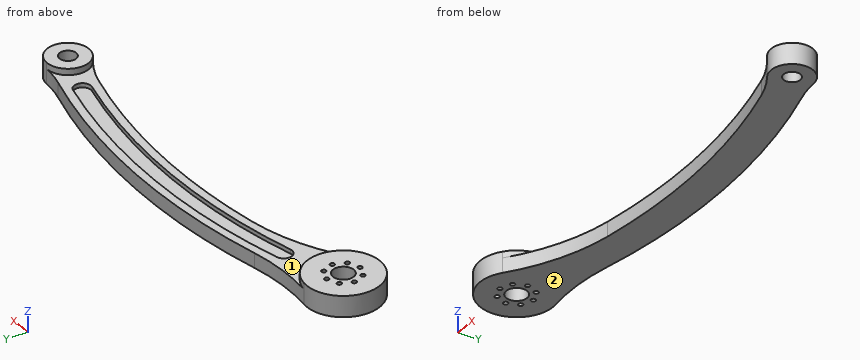
from build123d import *

# Parameters (mm, degrees)
SKETCH1_R                = 5
SKETCH1_R_2              = 4
BOSS_EXTRUDE1_DEPTH      = 10
FILLET1_R                = 100
FILLET3_R                = 50
BOSS_EXTRUDE2_DEPTH      = 5
CUT_EXTRUDE1_DEPTH       = 3
M2_CLEARANCE_HOLE2_D     = 2.2
M2_CLEARANCE_HOLE2_DEPTH = 10


with BuildPart() as part:
    # Sketch1 → Boss-Extrude1 (new body)
    with BuildSketch(Plane.XY):
        with BuildLine():
            ThreePointArc((12.332289397, 12.416305338), (-16.645203494, -5.40251799), (17.2733755, -2.807222621))
            ThreePointArc((17.2733755, -2.807222621), (104.699737116, 9.220908362), (191.757044964, -5.238337488))
            ThreePointArc((191.757044964, -5.238337488), (209.474645485, -2.773362317), (196.872940476, 9.922562291))
            ThreePointArc((196.872940476, 9.922562291), (104.792499107, 25.221141559), (12.332289397, 12.416305338))
        make_face()
        Circle(SKETCH1_R, mode=Mode.SUBTRACT)
        with Locations((199.999550741, 0.423914585)):
            Circle(SKETCH1_R_2, mode=Mode.SUBTRACT)
        with BuildLine():
            ThreePointArc((30.935149345, 4.991193321), (105.08187222, 13.215793431), (178.947951069, 2.766728612))
            ThreePointArc((178.947951069, 2.766728612), (183.85884318, 5.57442138), (181.051150412, 10.485313491))
            ThreePointArc((181.051150412, 10.485313491), (105.20208958, 21.214890117), (29.064850655, 12.769495373))
            ThreePointArc((29.064850655, 12.769495373), (26.110848974, 7.945195001), (30.935149345, 4.991193321))
        make_face(mode=Mode.SUBTRACT)
    extrude(amount=BOSS_EXTRUDE1_DEPTH)

    # Fillet1
    fillet1_edges = [part.edges().sort_by_distance(p)[0] for p in [
        (17.2733755, -2.807222621, 5),
        (12.332289397, 12.416305338, 5),
    ]]
    fillet(fillet1_edges, radius=FILLET1_R)

    # Fillet3
    fillet3_edges = [part.edges().sort_by_distance(p)[0] for p in [
        (196.872940476, 9.922562291, 5),
        (191.757044964, -5.238337488, 5),
    ]]
    fillet(fillet3_edges, radius=FILLET3_R)

    # Sketch2 → Boss-Extrude2 (add)
    with BuildSketch(Plane(origin=(0, 0, 0), x_dir=(-1, 0, 0), z_dir=(0, 0, -1))):
        with BuildLine():
            ThreePointArc((-30.935149345, 4.991193321), (-26.110848974, 7.945195001), (-29.064850655, 12.769495373))
            ThreePointArc((-29.064850655, 12.769495373), (-105.20208958, 21.214890117), (-181.051150412, 10.485313491))
            ThreePointArc((-181.051150412, 10.485313491), (-183.85884318, 5.57442138), (-178.947951069, 2.766728612))
            ThreePointArc((-178.947951069, 2.766728612), (-105.08187222, 13.215793431), (-30.935149345, 4.991193321))
        make_face()
    extrude(amount=-BOSS_EXTRUDE2_DEPTH)

    # Sketch3 → Cut-Extrude1 (cut)
    with BuildSketch(Plane.XY.offset(10)):
        with BuildLine():
            ThreePointArc((10.719889508, -13.832352256), (16.904607487, 4.525952466), (2.374455951, 17.338164809))
            ThreePointArc((2.374455951, 17.338164809), (19.536178227, 16.477975853), (36.591800033, 18.568526337))
            ThreePointArc((36.591800033, 18.568526337), (113.1236291, 24.996521405), (188.887012749, 12.412814518))
            ThreePointArc((188.887012749, 12.412814518), (194.644535138, 11.067035799), (200.520666376, 10.410327279))
            ThreePointArc((200.520666376, 10.410327279), (190.475667826, 3.472792121), (194.624244359, -8.008527607))
            ThreePointArc((194.624244359, -8.008527607), (188.279056755, -4.580565267), (181.506715916, -2.10110341))
            ThreePointArc((181.506715916, -2.10110341), (119.798948798, 8.622149082), (57.220022333, 6.030888954))
            ThreePointArc((57.220022333, 6.030888954), (32.693746361, -0.913106752), (10.719889508, -13.832352256))
        make_face()
    extrude(amount=-CUT_EXTRUDE1_DEPTH, mode=Mode.SUBTRACT)

    # M2 Clearance Hole2
    with Locations(Plane.XY.offset(10)):
        with Locations((0, 8), (5.656854249, 5.656854249), (8, 0), (5.656854249, -5.656854249), (0, -8), (-5.656854249, -5.656854249), (-8, 0), (-5.656854249, 5.656854249)):
            Hole(M2_CLEARANCE_HOLE2_D / 2, depth=M2_CLEARANCE_HOLE2_DEPTH)


solid = part.part
For this review, take the finished solid that the model builds, in its own axes (mm). Face numbers are marked on the shaded views. Round coordinates to 2 decimals unless told otherwise and drop trailing zeros. Order: outer loops, then holes, each group sorted by start corner. A loop starts at its lowest first (then second) coordinate and runs counter-clockwise, first axis right, second up. Notation, with made-up numbers: (-26, -9.5) -> (4, -9.5) arc R16 ccw to (4, 6.5) -> close; hole circle Ø10 at (26.5, -20.5). An arc over 180 degrees is marked (long way). Put each result on its own line as item: value.
Q1. Add section B-B on z = 2.75. State how many separate pieces and enclosed holes the cut face has, plus the area to 3 significant figures.
Check result:
separate pieces: 1
enclosed holes: 10
area: 4,110 mm2
Q2. Insertion check: pin 1 Ø1.5 at (x, z) = (146, 1.5) entering from -Y; pin 2 Ø1.8 at (x, y) = (-8, 0) entering from +Z; pin 3 Ø5 at (x, z) = (71.5, 4) entering from -Y; pin 4 Ø2 at (x, z) = (166.5, 5) entering from +Y. Each pin has a flat end and moves straight along its axis. Give the tip position at first contact, or say it passes through.
Check result:
pin 1: y = 5.61
pin 2: through
pin 3: y = 7.55
pin 4: y = 18.38
Q3. Add section A-A on x = 88.5. Write out the cut boundary in (y, z), plus the area to 3 significant figures.
Check result:
outline: (9, 0) -> (25.01, 0) -> (25.01, 7) -> (21.01, 7) -> (21.01, 5) -> (13, 5) -> (13, 7) -> (9, 7) -> close
area: 96.1 mm2
Q4. Mouldability with a two-part tool opening along X and no side actions: class the marked faces 1 and 2 as pulls with the +X half, pulls with the -X half, needs draft (parallel to the pull), parting line crosses it, or undercut.
Check result:
face 1: undercut
face 2: needs draft
Q5. Add section C-C on x = 115.5. Write out the cut boundary in (y, z), plus the area to 3 significant figures.
Check result:
outline: (8.87, 0) -> (24.89, 0) -> (24.89, 7) -> (20.89, 7) -> (20.89, 5) -> (12.88, 5) -> (12.88, 7) -> (8.87, 7) -> close
area: 96.1 mm2
Q6. For probe 1 along X at (y, z) = (-7, 4.5); probe 2 along Z at (x, y) = (148, 11.5); probe 3 along X at (y, z) = (7.5, 9), list the stretches that pass through material, from the lowest coordinate up. Write a range as [from, to].
Check result:
probe 1: [-16.04, -0.46], [0.46, 20.74], [192.97, 206.7]
probe 2: [0, 5]
probe 3: [-15.81, -0.98], [0.98, 15.81], [192.93, 207.07]
